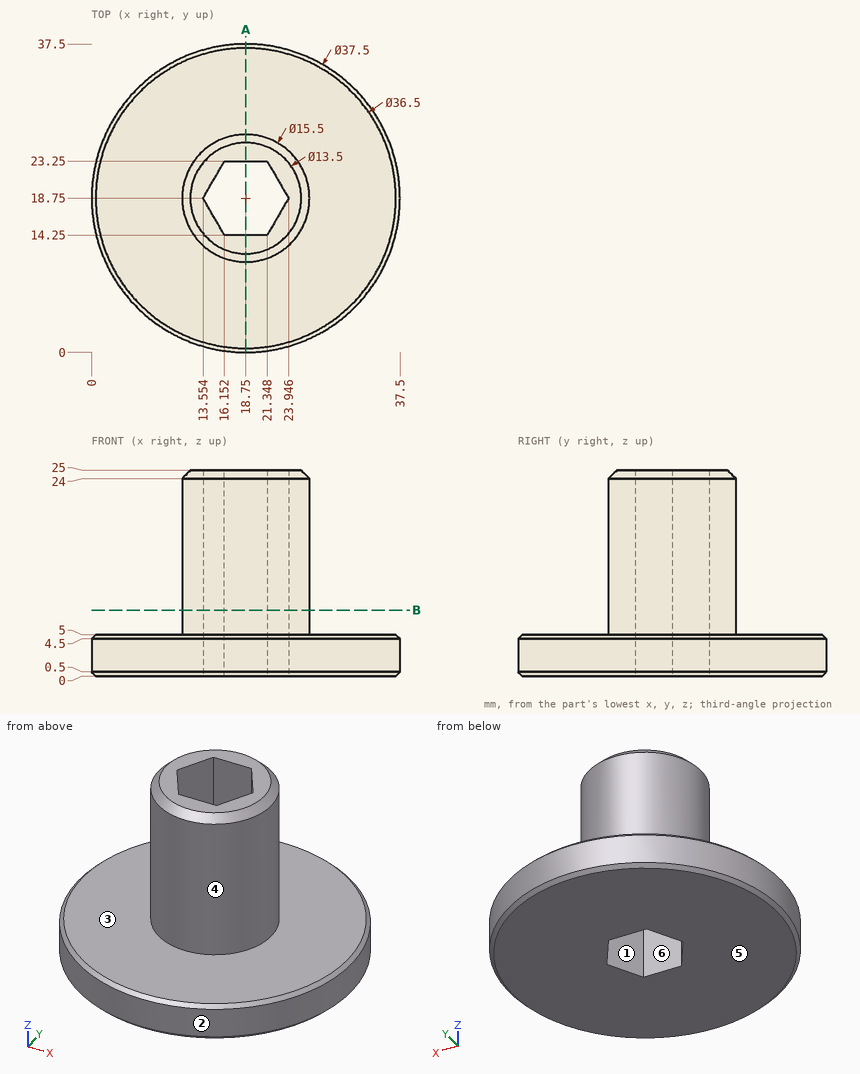
Here's the drawing with two shaded views (mm, measured from the low corner). I have some questions. A direction names the side the tool comes from. Give positions to 0.01 mm unless a question says otherwise; leave off trailing zeros. Loops run counter-clockwise (first coordinate to the right, second up) from the corner with the lowest first, then second, coordinate; pieces in that order, holes last. Notation, with made-up numbers: (25.25, 31) -> (61.25, 31) arc R22 ccw to (61.25, 70) -> close; hole circle Ø11 at (-40, 9.25). An arc over 180 degrees is marked (long way). Use one line per item in the form item = value.
1) For the marked faces 4, 5 and 6, which set-ups out of +Z, -Z, +X, -X, +Y, -Y let a thin tool reach every point of the face, with its end or its side?
Answers:
face_4 = +Z
face_5 = -Z, +X, -X, +Y, -Y
face_6 = +Z, -Z
2) Will these pins go through, and if not, where does the flat tip stop? pin 1 (4 mm diameter, centred on y = 30, z = 21.5, fed in from -X); pin 2 (10 mm diameter, centred on y = 17.5, z = 19.5, fed in from +X); pin 3 (1 mm diameter, centred on x = 19.5, z = 12, fed in from -Y); pin 4 (6 mm diameter, centred on x = 11, y = 31, fed in from +Z).
Answers:
pin_1 = through
pin_2 = 26.5
pin_3 = 11
pin_4 = 5
3) We'd pull the mould along Y, two halves only. Please class the marked faces 1, 2 and 3: released by +Y, released by -Y, zero draft, split by the parting line, or undercut.
Answers:
face_1 = undercut
face_2 = split by the parting line
face_3 = zero draft
4) I need wall thicknesses on line 1 along X through (y, z) = (24.5, 21.5); line 2 along Z through (x, y) = (30, 30.5); line 3 along Y through (x, z) = (18, 22.25). Which ranges of each line are inside material? Lowest first, please.
Answers:
line_1 = 13.55 to 23.95
line_2 = 0 to 5
line_3 = 11.04 to 14.25, 23.25 to 26.46
5) If we section it at A-A (x = 18.75): Please give me the cut outline in (y, z), plus the area to 3 significant figures.
Answers:
outline = (0, 0.5) -> (0.5, 0) -> (14.25, 0) -> (14.25, 25) -> (12, 25) -> (11, 24) -> (11, 5) -> (0.5, 5) -> (0, 4.5) -> close; (23.25, 0) -> (37, 0) -> (37.5, 0.5) -> (37.5, 4.5) -> (37, 5) -> (26.5, 5) -> (26.5, 24) -> (25.5, 25) -> (23.25, 25) -> close
area = 271 mm²
6) If we section it at B-B (z = 8): Please give me the cut outline in (x, y).
Answers:
outline = circle Ø15.5 at (18.75, 18.75); hole (13.55, 18.75) -> (16.15, 14.25) -> (21.35, 14.25) -> (23.95, 18.75) -> (21.35, 23.25) -> (16.15, 23.25) -> close
